Geometry: final body of the model. Coordinates: model frame, mm. A direction names the side the tool comes from. Coordinates: 2 decimals unless noted, no trailing zeros. Order: outer loops, then holes, each group sorted by start corner. A loop starts at its lowest first (then second) coordinate and runs counter-clockwise, first axis right, second up. Notation, with made-up numbers: M 67,3.5 L 110,3.5 A24 ccw 110,36.5 Z; hole C 62,-2 d8. An arc over 180 degrees is marked long. Use CSV: the item, a comma, the result in double quotes. Start each with the question number.
1. Section query D-D on z = 2.15. Return the cut outline in (x, y).
2. Material intervals for line 1 (X direction, y = -0.5, z = 1.65); line 2 (Y direction, x = 0.5, z = 1.75); line 3 (Y direction, x = -2, z = 1.85), sorted ascending.
3. First-contact query: P1, Ø1.5, axis at x = -1, z = 2, coming from the +Y side; P2, Ø2, axis at x = 0.5, z = 1, coming from the +Y side; P3, Ø0.7, axis at y = 1, z = 1.5, coming from the +X side; P4, Ø1.5, axis at y = 0.5, z = -1, coming from the +X side. Flat tips, straight axial feed; report the tip coordinate or a pass-through.
4. Section query B-B on x = 0. Return the cut outline in (y, z), and give its area (3 significant figures).
5. Set-up query: faces 5 (the flat face through (0, 2.5, 2)), 6 (the flat face through (2.25, 0, 2)), 7 (the flat face through (1.05, 0, 1)), 8 (the flat face through (-2, 0, 2.4)), 9 (the flat face through (-2.25, 0, 2)). Return all of +Z, -Z, +X, -X, +Y, -Y with unobstructed straight access to the full face (end or side cutting, diameter ignored); none if empty.
6. Pull-direction query (X, two-part tool) for faces 1 (the flat face through (0, 1.3, 1)), 2 (the cylindrical face through (-5.994, 0.264, 0.197)), 3 (the flat face through (0, -2.5, 2)), 4 (the flat face through (0, -1.3, 1)); classes: pulls with the +X half, pulls with the -X half, needs draft (parallel to the pull), parting line crosses it, or undercut.
7. Section query A-A on z = 0.6. Return the cut outline in (x, y).
8. Section query C-C on y = 2. Return the cut outline in (x, z).
from build123d import *

# Parameters (mm, degrees)
ESQUISSE1_R        = 6
BOSS_EXTRU_1_DEPTH = 0.4
D_ME1_FACE_RADIUS  = 6
D_ME1_HEIGHT       = 1.8
ESQUISSE3_W        = 4.5
ESQUISSE3_H        = 5
ESQUISSE3_W_2      = 2.1
ESQUISSE3_H_2      = 2.6
EXTRU_MINCE1_DEPTH = 2
CHANFREIN1_SIZE    = 0.6


with BuildPart() as part:
    # Esquisse1 → Boss.-Extru.1 (new body)
    with BuildSketch(Plane.XY):
        Circle(ESQUISSE1_R)
    extrude(amount=BOSS_EXTRU_1_DEPTH)

    # Dôme1: a dome of height H over a round flat face of radius A is a cap of a sphere of radius (A * A + H * H) / (2 * H)
    d_me1_r = (D_ME1_FACE_RADIUS * D_ME1_FACE_RADIUS + D_ME1_HEIGHT * D_ME1_HEIGHT) / (2 * D_ME1_HEIGHT)
    d_me1_base = Plane((0, 0, 0), z_dir=(0, 0, -1))
    with Locations(d_me1_base.offset(D_ME1_HEIGHT - d_me1_r)):
        d_me1_ball = Sphere(d_me1_r, mode=Mode.PRIVATE)
    add(split(d_me1_ball, bisect_by=d_me1_base, keep=Keep.TOP, mode=Mode.PRIVATE))

    # Esquisse3 → Extru.-Mince1 (add)
    with BuildSketch(Plane.XY.offset(0.4)):
        Rectangle(ESQUISSE3_W, ESQUISSE3_H)
        Rectangle(ESQUISSE3_W_2, ESQUISSE3_H_2, mode=Mode.SUBTRACT)
    extrude(amount=EXTRU_MINCE1_DEPTH)

    # Chanfrein1
    chanfrein1_edges = [part.edges().sort_by_distance(p)[0] for p in [
        (2.25, 0, 0.4),
        (0, 2.5, 0.4),
        (-2.25, 0, 0.4),
        (0, -2.5, 0.4),
    ]]
    chamfer(chanfrein1_edges, length=CHANFREIN1_SIZE)


solid = part.part
Results list:
1,outline,"M -2.25,-2.5 L 2.25,-2.5 L 2.25,2.5 L -2.25,2.5 Z; hole M -1.05,-1.3 L 1.05,-1.3 L 1.05,1.3 L -1.05,1.3 Z"
2,line 1,"x = -2.25 to -1.05, 1.05 to 2.25"
2,line 2,"y = -2.5 to -1.3, 1.3 to 2.5"
2,line 3,"y = -2.5 to 2.5"
3,P1,"stops at y = 2.5"
3,P2,"stops at y = 6"
3,P3,"stops at x = 2.25"
3,P4,"stops at x = 5.58"
4,outline,"M -6,0 A10.9 ccw 6,0 L 6,0.4 L 3.1,0.4 L 2.5,1 L 2.5,2.4 L 1.3,2.4 L 1.3,0.4 L -1.3,0.4 L -1.3,2.4 L -2.5,2.4 L -2.5,1 L -3.1,0.4 L -6,0.4 Z"
4,area,"24.6 mm²"
5,face 5,"+Z, +X, -X, +Y"
5,face 6,"+Z, +X, +Y, -Y"
5,face 7,"+Z"
5,face 8,"+Z, +X, -X, +Y, -Y"
5,face 9,"+Z, -X, +Y, -Y"
6,face 1,"undercut"
6,face 2,"parting line crosses it"
6,face 3,"needs draft"
6,face 4,"undercut"
7,outline,"M -2.65,-2.9 L 2.65,-2.9 L 2.65,2.9 L -2.65,2.9 Z; hole M -1.05,-1.3 L 1.05,-1.3 L 1.05,1.3 L -1.05,1.3 Z"
8,outline,"M -5.66,0 A10.71 ccw 5.66,0 L 5.66,0.4 L 2.85,0.4 L 2.25,1 L 2.25,2.4 L -2.25,2.4 L -2.25,1 L -2.85,0.4 L -5.66,0.4 Z"
